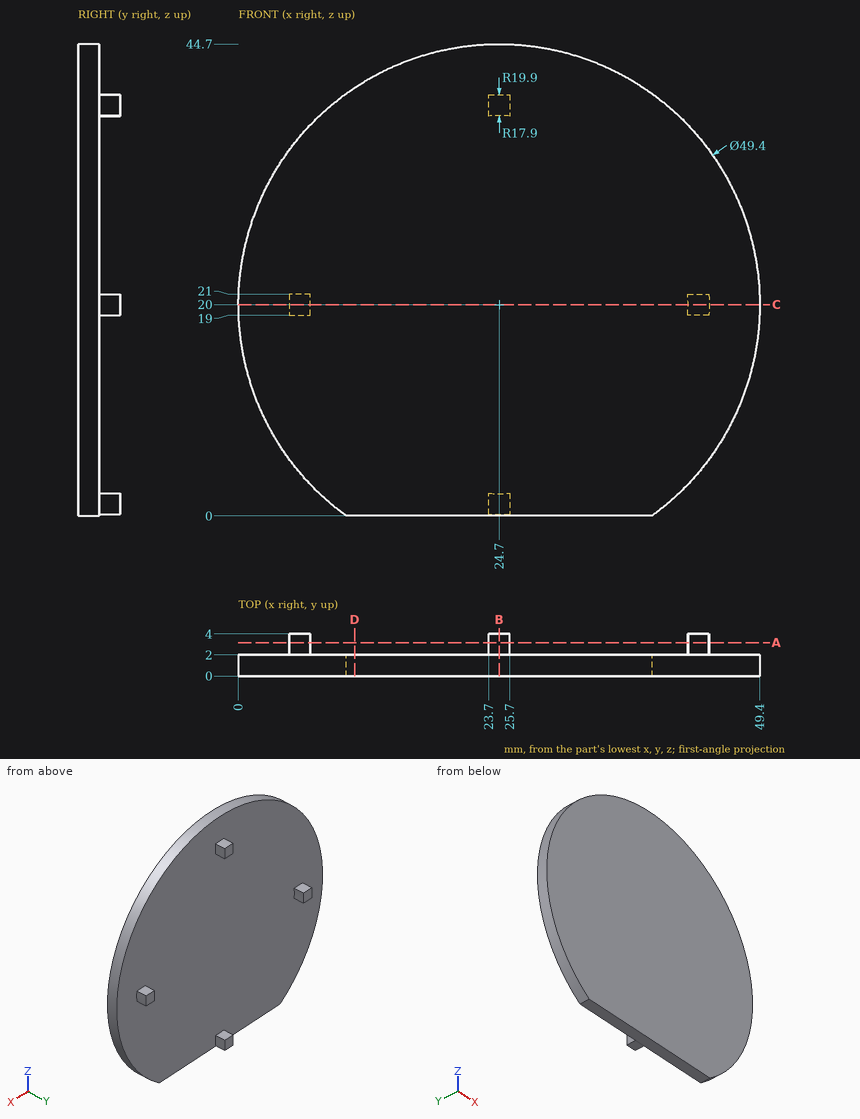
Could you check a few things on this drawing? It's one solid part, dimensions in mm from its lowest x, y, z. Coordinates: 2 decimals unless noted, no trailing zeros. Loops run counter-clockwise (first coordinate to the right, second up) from the corner with the lowest first, then second, coordinate; pieces in that order, holes last.
1. Imagine slicing it at D-D (x = 11). Please give me the cut outline in (y, z), and give its area (3 significant figures).
2. For P1, Ø0.6, axis at x = 43, y = 2.5, coming from the +Z side; P2, Ø1.6, axis at x = 6.5, y = 3, coming from the -Z side; P3, Ø2, axis at x = 43.5, y = 2.5, coming from the -Z side; P4, Ø5, axis at x = 16, z = 19.5, coming from the -Y side, each with a flat end and sliding along its axis, tell me the tip position at first contact or that it passes through.
3. I need wall thicknesses on L1, parallel to Y at x = 10, z = 17.5; L2, parallel to X at y = 3.7, z = 38.5; L3, parallel to Z at x = 11.5, y = 1. Which ranges of each line are inside material? Lowest first, please.
4. Imagine slicing it at C-C (z = 20). Please give me the cut outline in (x, y).
5. Imagine slicing it at A-A (y = 3.15). Please give me the cut outline in (x, z).
6. Imagine slicing it at B-B (x = 24.7). Please give me the cut outline in (y, z).
Computed values:
1. outline: (0, 0) - (2, 0) - (2, 40.55) - (0, 40.55) - close
1. area: 81.1 mm2
2. P1: stops at z = 21
2. P2: stops at z = 19
2. P3: stops at z = 3.02
2. P4: stops at y = 0
3. L1: y = 0 to 2
3. L2: x = 23.7 to 25.7
3. L3: z = 0 to 40.88
4. outline: (0, 0) - (49.4, 0) - (49.4, 2) - (44.6, 2) - (44.6, 4) - (42.6, 4) - (42.6, 2) - (6.8, 2) - (6.8, 4) - (4.8, 4) - (4.8, 2) - (0, 2) - close
5. outline: (4.83, 19) - (6.83, 19) arc R17.9 cw to (6.83, 21) - (4.83, 21) arc R19.9 ccw to start; (23.7, 0.13) arc R19.9 ccw to (25.7, 0.13) - (25.7, 2.13) arc R17.9 cw to (23.7, 2.13) - close; (23.7, 37.87) arc R17.9 cw to (25.7, 37.87) - (25.7, 39.87) arc R19.9 ccw to (23.7, 39.87) - close; (42.57, 19) - (44.57, 19) arc R19.9 ccw to (44.57, 21) - (42.57, 21) arc R17.9 cw to start
6. outline: (0, 0) - (2, 0) - (2, 0.1) - (4, 0.1) - (4, 2.1) - (2, 2.1) - (2, 37.9) - (4, 37.9) - (4, 39.9) - (2, 39.9) - (2, 44.7) - (0, 44.7) - close
